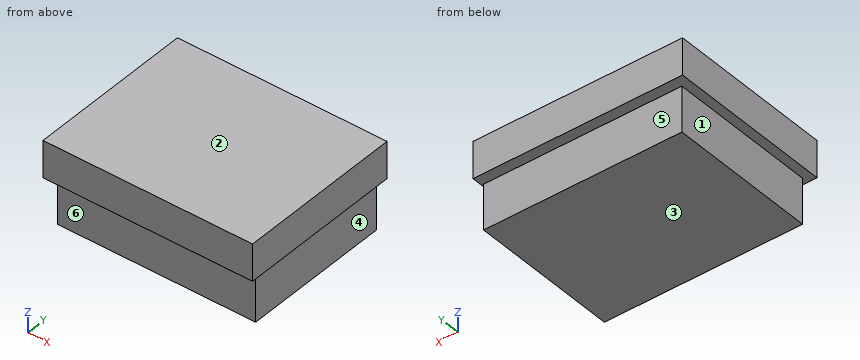
from build123d import *

# Parameters (mm, degrees)
F0_W      = 74
F0_H      = 59
F1_DEPTH  = 13
F2_W      = 70
F2_H      = 53
F3_DEPTH  = 3
F3_FACE_W = 70
F3_FACE_H = 53
F4_DEPTH  = 13


with BuildPart() as f1:
    # F0 (on Top) → F1 (new body)
    with BuildSketch(Plane.XY):
        with Locations((-86.124225, -25.756026)):
            Rectangle(F0_W, F0_H)
    extrude(amount=F1_DEPTH)

    # F2 (on Top) → F3 (join)
    with BuildSketch(Plane.XY):
        with Locations((-84.860367, -26.5)):
            Rectangle(F2_W, F2_H)
    extrude(amount=-F3_DEPTH)

    # F3_face (on face) → F4 (join)
    with BuildSketch(Plane(origin=(-84.860367, -26.5, -3), x_dir=(1, 0, 0), z_dir=(0, 0, -1))):
        Rectangle(F3_FACE_W, F3_FACE_H)
    extrude(amount=F4_DEPTH)


solid = f1.part
Part model, mm, in its own coordinate system. Face numbers are marked on the shaded views. A direction names the side the tool comes from. Coordinates: 2 decimals unless noted, no trailing zeros. Loops run counter-clockwise (first coordinate to the right, second up) from the corner with the lowest first, then second, coordinate; pieces in that order, holes last. Notation, with made-up numbers: M -2.75,71 L 7.25,71 A38 cw 7.25,110 Z; hole C 85,85.5 d5. An arc over 180 degrees is marked long. Use a Markdown table: item, result. Add a question column.
Q1. Cut at C-C (z = -6.25). Write the cut outline in (x, y).
Q2. Probe L1, parallel to X at y = -29.5, z = -7.75; L2, parallel to Y at x = -112, z = -10.75. List the from-to ranges inside material, lowest first.
Q3. Mould opens along Z. For the marked faces 1, 2 and 3 say: +Z half, -Z half, draft (parallel to the pull), parting line (faces both ways), or undercut.
Q4. Cut at A-A (x = -99). Write the cut outline in (y, z).
Q5. Which spindle directions (+Z, -Z, +X, -X, +Y, -Y) get a long thin tool onto all of the face, cutting with end or side? Do the marked faces 4, 5 and 6. Say none if no direction does.
Q6. Pin check, flat tips, straight feed: P1, Ø8, axis at x = -76, z = -12, coming from the -Y side; P2, Ø8, axis at x = -97.5, z = -10.5, coming from the +Y side; P3, Ø8, axis at y = -39, z = -11, coming from the -X side. Stop position of each tip, or through.
Q7. Cut at B-B (y = -37). Write the cut outline in (x, z), and give its area (3 significant figures).
Worked out:
| question | item | result |
|---|---|---|
| 1 | outline | M -119.86,-53 L -49.86,-53 L -49.86,0 L -119.86,0 Z |
| 2 | L1 | x = -119.86 to -49.86 |
| 2 | L2 | y = -53 to 0 |
| 3 | face 1 | draft |
| 3 | face 2 | +Z half |
| 3 | face 3 | -Z half |
| 4 | outline | M -55.26,0 L -53,0 L -53,-16 L 0,-16 L 0,0 L 3.74,0 L 3.74,13 L -55.26,13 Z |
| 5 | face 4 | -Z, +X, +Y, -Y |
| 5 | face 5 | -Z, +X, -X, +Y |
| 5 | face 6 | -Z, +X, -X, -Y |
| 6 | P1 | stops at y = -53 |
| 6 | P2 | stops at y = 0 |
| 6 | P3 | stops at x = -119.86 |
| 7 | outline | M -123.12,0 L -119.86,0 L -119.86,-16 L -49.86,-16 L -49.86,0 L -49.12,0 L -49.12,13 L -123.12,13 Z |
| 7 | area | 2,080 mm2 |
